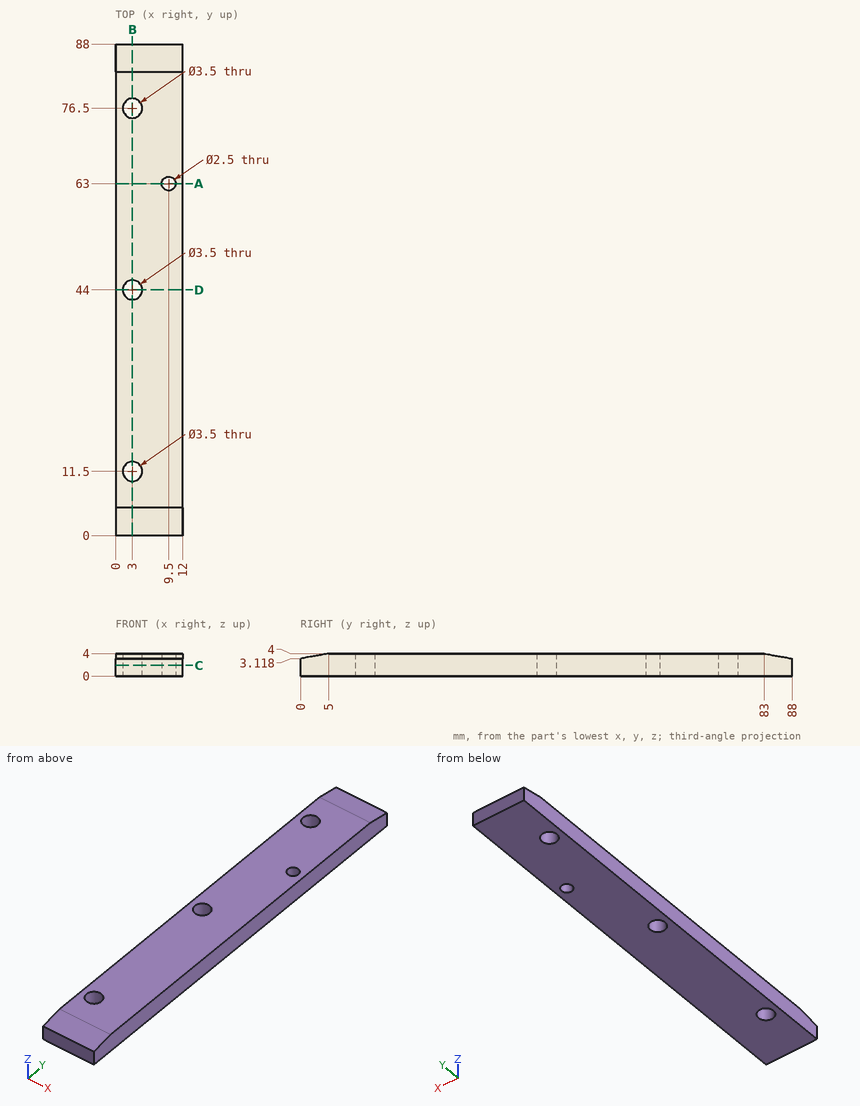
For this review, use the dimensioned drawing (mm, ordinates from the lowest corner) and the shaded views. Coordinates: 2 decimals unless noted, no trailing zeros. Write each loop counter-clockwise with the first axis right and the second up, starting at its lowest first coordinate (ties: lowest second). Pieces come first, ordered by that corner, then holes. Notation, with made-up numbers: (74.5, 23.5) -> (131.5, 23.5) arc R28 ccw to (131.5, 42.5) -> close; hole circle Ø2 at (68.25, 24). An arc over 180 degrees is marked (long way). Write each question's results on one line, items separated by ' | '. Start each with the question number.
(1) Take a section at A-A on y = 63. Write out the cut boundary in (x, z), and give its area (3 significant figures).
(2) Clearance check with a flat-ended pin moving along its axis: P1, Ø1.5, axis at x = 5, z = 0.5, coming from the -Y side. State where the tip first meets the part, or that it passes through.
(3) Take a section at B-B on x = 3. Write out the cut boundary in (y, z).
(4) Take a section at C-C on z = 1.9. Write out the cut boundary in (x, y), and give its area (3 significant figures).
(5) For line 1 along Y through (x, z) = (3, 1.5); line 2 along X through (y, z) = (11.5, 1.05); line 3 along Y through (x, z) = (4, 1.05) (1 decimal), list the stretches that pass through material, from the lowest coordinate up. Write a range as from..to.
(6) Take a section at D-D on y = 44. Write out the cut boundary in (x, z).
Results found:
1) outline: (0, 0) -> (8.25, 0) -> (8.25, 4) -> (0, 4) -> close; (10.75, 0) -> (12, 0) -> (12, 4) -> (10.75, 4) -> close | area: 38.0 mm2
2) P1: stops at y = 0
3) outline: (0, 0) -> (9.75, 0) -> (9.75, 4) -> (5, 4) -> (0, 3.12) -> close; (13.25, 0) -> (42.25, 0) -> (42.25, 4) -> (13.25, 4) -> close; (45.75, 0) -> (74.75, 0) -> (74.75, 4) -> (45.75, 4) -> close; (78.25, 0) -> (88, 0) -> (88, 3.12) -> (83, 4) -> (78.25, 4) -> close
4) outline: (0, 0) -> (12, 0) -> (12, 88) -> (0, 88) -> close; hole circle Ø3.5 at (3, 11.5); hole circle Ø3.5 at (3, 44); hole circle Ø3.5 at (3, 76.5); hole circle Ø2.5 at (9.5, 63) | area: 1,020 mm2
5) line 1: y = 0..9.75, 13.25..42.25, 45.75..74.75, 78.25..88 | line 2: x = 0..1.25, 4.75..12 | line 3: y = 0..10.1, 12.9..42.6, 45.4..75.1, 77.9..88
6) outline: (0, 0) -> (1.25, 0) -> (1.25, 4) -> (0, 4) -> close; (4.75, 0) -> (12, 0) -> (12, 4) -> (4.75, 4) -> close
